Model file for the job. Use its own axes, mm. Face numbers are marked on the shaded views. A direction names the side the tool comes from. Round coordinates to 2 decimals unless told otherwise and drop trailing zeros. Order: outer loops, then holes, each group sorted by start corner. A loop starts at its lowest first (then second) coordinate and runs counter-clockwise, first axis right, second up. Notation, with made-up numbers: (25.5, 33) -> (46.5, 33) arc R14 ccw to (46.5, 43) -> close; hole circle Ø10 at (52.5, 89.25). An arc over 180 degrees is marked (long way). Put each result on its own line as item: value. Start each with the question number.
Q1. Pull direction Y, two halves, no side cores. Call the marked faces 1, 2, 3 and 4: released by +Y, released by -Y, zero draft, split by the parting line, or undercut.
Q2. 3-axis set-ups, long thin cutter, end or side, ignore diameter. For the marked faces 5, 6, 7, 8 and 9: which of +Z, -Z, +X, -X, +Y, -Y reach the whole face in a straight line?
Q3. Cut at C-C, the plane z = 2. List the corners of the cut face in (x, y).
Q4. Cut at A-A, the plane z = -7.25. List the corners of the cut face in (x, y), and give its area (3 significant figures).
Q5. Probe L1, parallel to Y at x = 12.5, z = 2.1; L2, parallel to Y at x = -10, z = 1.5; L3, parallel to X at y = 19, z = -7.75. List the from-to ranges inside material, lowest first.
Q6. Cut at D-D, the plane x = 42.5. List the corners of the cut face in (y, z), and give its area (3 significant figures).
Q7. Flat gauge pins, fed straight in: P1, Ø3.5, axis at x = -10, y = 47.5, coming from the -Z side; P2, Ø7, axis at x = 12.5, y = 70, coming from the -Z side; P3, Ø1.2, axis at x = 12.5, z = 6, coming from the -Y side; P4, Ø2, axis at y = 45, z = 3, coming from the +X side. Where does each tip first touch, or does it go through?
Q8. Cut at B-B, the plane x = -10. List the corners of the cut face in (y, z).
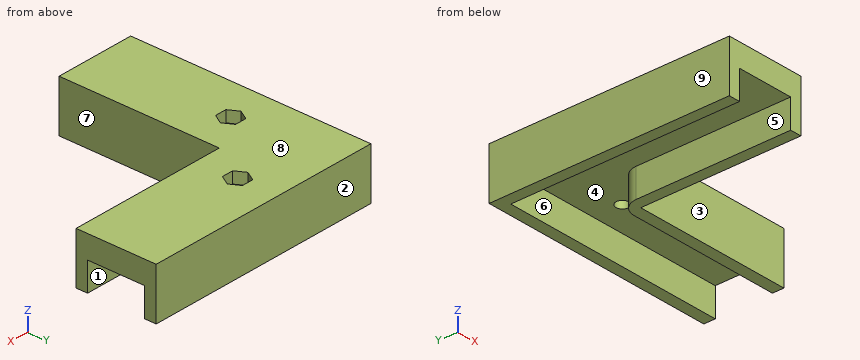
from build123d import *

# Parameters (mm, degrees)
BOSS_EXTRU_1_DEPTH      = 8
ENL_V_MAT_EXTRU_1_DEPTH = 4
ESQUISSE3_R             = 2.25
ENL_V_MAT_EXTRU_2_DEPTH = 5
BOSS_EXTRU_2_DEPTH      = 18
CONG_1_R                = 6


with BuildPart() as part:
    # Esquisse1 → Boss.-Extru.1 (new body)
    with BuildSketch(Plane.XY):
        Polygon((0, 0), (0, 60), (60, 60), (60, 80), (-20, 80), (-20, 0), align=None)
    extrude(amount=BOSS_EXTRU_1_DEPTH)

    # Esquisse2 → Enlèv. mat.-Extru.1 (cut)
    with BuildSketch(Plane.XY.offset(8)):
        Polygon((-14.041451884, 47.5), (-12.020725942, 51), (-7.979274058, 51), (-5.958548116, 47.5), (-7.979274058, 44), (-12.020725942, 44), align=None)
        Polygon((8.458548116, 70), (10.479274058, 73.5), (14.520725942, 73.5), (16.541451884, 70), (14.520725942, 66.5), (10.479274058, 66.5), align=None)
    extrude(amount=-ENL_V_MAT_EXTRU_1_DEPTH, mode=Mode.SUBTRACT)

    # Esquisse3 → Enlèv. mat.-Extru.2 (cut, through all)
    with BuildSketch(Plane.XY.offset(4)):
        with Locations((-10, 47.5)):
            Circle(ESQUISSE3_R)
        with Locations((12.5, 70)):
            Circle(ESQUISSE3_R)
    extrude(amount=-ENL_V_MAT_EXTRU_2_DEPTH, mode=Mode.SUBTRACT)

    # Esquisse4 → Boss.-Extru.2 (add)
    with BuildSketch(Plane.XY.offset(8)):
        Polygon((0, 0), (0, 60), (60, 60), (60, 56), (4, 56), (4, 0), align=None)
        Polygon((60, 80), (60, 84), (-24, 84), (-24, 0), (-20, 0), (-20, 80), align=None)
    extrude(amount=-BOSS_EXTRU_2_DEPTH)

    # Congé1
    cong_1_edges = [part.edges().sort_by_distance(p)[0] for p in [
        (0, 60, -5),
    ]]
    fillet(cong_1_edges, radius=CONG_1_R)


solid = part.part
Ans:
1. face 1: undercut
1. face 2: released by +Y
1. face 3: released by -Y
1. face 4: undercut
2. face 5: -Z, -Y
2. face 6: -Z, +X
2. face 7: +Z, -Z, +X, -Y
2. face 8: +Z, +X, -X, +Y, -Y
2. face 9: +Z, -Z, -X, +Y, -Y
3. outline: (-24, 0) -> (4, 0) -> (4, 56) -> (60, 56) -> (60, 84) -> (-24, 84) -> close; hole circle Ø4.5 at (-10, 47.5); hole circle Ø4.5 at (12.5, 70)
4. outline: (-24, 0) -> (-20, 0) -> (-20, 80) -> (60, 80) -> (60, 84) -> (-24, 84) -> close; (0, 0) -> (4, 0) -> (4, 56) -> (60, 56) -> (60, 60) -> (6, 60) arc R6 ccw to (0, 54) -> close
4. area: 1,110 mm^2
5. L1: y = 56 to 67.75, 72.25 to 84
5. L2: y = 0 to 45.25, 49.75 to 84
5. L3: x = -24 to -20, 0 to 4
6. outline: (56, -10) -> (60, -10) -> (60, 0) -> (80, 0) -> (80, -10) -> (84, -10) -> (84, 8) -> (56, 8) -> close
6. area: 304 mm^2
7. P1: passes through
7. P2: stops at z = 0
7. P3: stops at y = 56
7. P4: stops at x = 4
8. outline: (0, 0) -> (45.25, 0) -> (45.25, 4) -> (44, 4) -> (44, 8) -> (0, 8) -> close; (49.75, 0) -> (80, 0) -> (80, -10) -> (84, -10) -> (84, 8) -> (51, 8) -> (51, 4) -> (49.75, 4) -> close
